```python
from build123d import *

# Parameters (mm, degrees)
SKETCH_1_R          = 4.5
SKETCH_1_R_2        = 1.5
SKETCH_1_W          = 5
SKETCH_1_H          = 9
SKETCH_1_R_3        = 2.5
SKETCH_1_R_4        = 1.1
EXTRUDE_1_DEPTH     = 3
CUT_EXTRUDE_1_DEPTH = 35.179672321


with BuildPart() as part:
    # 草图1 → 凸台-拉伸1 (new body)
    # profile 1 of 12: a face of its own
    with BuildSketch(Plane(origin=(0, 0, 0), x_dir=(1, 0, 0), z_dir=(0, 1, 0))):
        with Locations((-25, 0)):
            Circle(SKETCH_1_R)
        with Locations(Location((-25, 0, 0), (0, 0, 270))):
            Circle(SKETCH_1_R_2, mode=Mode.SUBTRACT)
    # profile 2 of 12: a face of its own
    with BuildSketch(Plane(origin=(0, 0, 0), x_dir=(1, 0, 0), z_dir=(0, 1, 0))):
        with BuildLine():
            Line((-18.5, 4.5), (-25, 4.5))
            ThreePointArc((-25, 4.5), (-21.818019485, 3.181980515), (-20.5, 0))
            ThreePointArc((-20.5, 0), (-21.818019485, -3.181980515), (-25, -4.5))
            Line((-25, -4.5), (-18.5, -4.5))
            Line((-18.5, -4.5), (-18.5, 4.5))
        make_face()
    # profile 3 of 12: a face of its own
    with BuildSketch(Plane(origin=(0, 0, 0), x_dir=(1, 0, 0), z_dir=(0, 1, 0))):
        with Locations((-16, 0)):
            Rectangle(SKETCH_1_W, SKETCH_1_H)
    # profile 4 of 12: a face of its own
    with BuildSketch(Plane(origin=(0, 0, 0), x_dir=(1, 0, 0), z_dir=(0, 1, 0))):
        with BuildLine():
            Line((-13.5, -4.5), (-18.5, -4.5))
            Line((-18.5, -4.5), (-18.5, -15.7))
            Line((-18.5, -15.7), (-7.000000018, -15.7))
            ThreePointArc((-7.000000018, -15.7), (-9.5, -13.199999991), (-7, -10.7))
            Line((-7, -10.7), (-13.5, -10.7))
            Line((-13.5, -10.7), (-13.5, -4.5))
        make_face()
    # profile 5 of 12: a face of its own
    with BuildSketch(Plane(origin=(0, 0, 0), x_dir=(1, 0, 0), z_dir=(0, 1, 0))):
        with BuildLine():
            Line((4.5, -4.5), (-0.5, -4.5))
            Line((-0.5, -4.5), (-0.5, -10.7))
            Line((-0.5, -10.7), (-7, -10.7))
            ThreePointArc((-7, -10.7), (-5.232233047, -11.432233047), (-4.5, -13.2))
            ThreePointArc((-4.5, -13.2), (-5.232233054, -14.967766959), (-7.000000018, -15.7))
            Line((-7.000000018, -15.7), (4.5, -15.7))
            Line((4.5, -15.7), (4.5, -4.5))
        make_face()
    # profile 6 of 12: a face of its own
    with BuildSketch(Plane(origin=(0, 0, 0), x_dir=(1, 0, 0), z_dir=(0, 1, 0))):
        Polygon((4.5, 4.5), (-0.5, 4.5), (-0.5, -4.5), (4.5, -4.5), (4.5, 0), align=None)
    # profile 7 of 12: a face of its own
    with BuildSketch(Plane(origin=(0, 0, 0), x_dir=(1, 0, 0), z_dir=(0, 1, 0))):
        with BuildLine():
            Line((-0.5, 12), (-0.5, 4.5))
            Line((-0.5, 4.5), (4.5, 4.5))
            Line((4.5, 4.5), (4.5, 17))
            Line((4.5, 17), (-7.000000057, 17))
            ThreePointArc((-7.000000057, 17), (-5.232233067, 16.267766973), (-4.5, 14.5))
            ThreePointArc((-4.5, 14.5), (-5.232233047, 12.732233047), (-7, 12))
            Line((-7, 12), (-0.5, 12))
        make_face()
    # profile 8 of 12: a face of its own
    with BuildSketch(Plane(origin=(0, 0, 0), x_dir=(1, 0, 0), z_dir=(0, 1, 0))):
        with BuildLine():
            Line((-18.5, 17), (-18.5, 4.5))
            Line((-18.5, 4.5), (-13.5, 4.5))
            Line((-13.5, 4.5), (-13.5, 12))
            Line((-13.5, 12), (-7, 12))
            ThreePointArc((-7, 12), (-9.5, 14.499999972), (-7.000000057, 17))
            Line((-7.000000057, 17), (-18.5, 17))
        make_face()
    # profile 9 of 12: a face of its own
    with BuildSketch(Plane(origin=(0, 0, 0), x_dir=(1, 0, 0), z_dir=(0, 1, 0))):
        with BuildLine():
            Line((25, 4.5), (4.5, 4.5))
            Line((4.5, 4.5), (4.5, 0))
            Line((4.5, 0), (4.5, -4.5))
            Line((4.5, -4.5), (25, -4.5))
            ThreePointArc((25, -4.5), (20.5, 0), (25, 4.5))
        make_face()
    # profile 10 of 12: a face of its own
    with BuildSketch(Plane(origin=(0, 0, 0), x_dir=(1, 0, 0), z_dir=(0, 1, 0))):
        with Locations((25, 0)):
            Circle(SKETCH_1_R)
        with Locations(Location((25, 0, 0), (0, 0, 270))):
            Circle(SKETCH_1_R_2, mode=Mode.SUBTRACT)
    # profile 11 of 12: a face of its own
    with BuildSketch(Plane(origin=(0, 0, 0), x_dir=(1, 0, 0), z_dir=(0, 1, 0))):
        with Locations((-7, 14.5)):
            Circle(SKETCH_1_R_3)
        with Locations(Location((-7, 14.5, 0), (0, 0, 270))):
            Circle(SKETCH_1_R_4, mode=Mode.SUBTRACT)
    # profile 12 of 12: a face of its own
    with BuildSketch(Plane(origin=(0, 0, 0), x_dir=(1, 0, 0), z_dir=(0, 1, 0))):
        with Locations((-7, -13.2)):
            Circle(SKETCH_1_R_3)
        with Locations(Location((-7, -13.2, 0), (0, 0, 270))):
            Circle(SKETCH_1_R_4, mode=Mode.SUBTRACT)
    extrude(amount=EXTRUDE_1_DEPTH)

    # 草图2 → 切除-拉伸1 (cut, through all)
    with BuildSketch(Plane(origin=(0, 3, 0), x_dir=(1, 0, 0), z_dir=(0, 1, 0))):
        Polygon((4.5, -15.7), (4.5, -11.296015474), (-4.064964363, -15.7), align=None)
    extrude(amount=-CUT_EXTRUDE_1_DEPTH, mode=Mode.SUBTRACT)


solid = part.part
```
Check sheet for the modelled part. Datum: model origin and axes. Units: mm. A direction names the side the tool comes from. Coordinates: 2 decimals unless noted, no trailing zeros. Write each loop counter-clockwise with the first axis right and the second up, starting at its lowest first coordinate (ties: lowest second). Pieces come first, ordered by that corner, then holes. Notation, with made-up numbers: (44, -16.75) -> (56, -16.75) arc R24 ccw to (56, 4.25) -> close; hole circle Ø5 at (37.5, 55.25). An arc over 180 degrees is marked (long way). Use a Markdown table: item, result.
1. Sectioned sample at C-C (x = -7). Enter the section's corners in (y, z), plus the area to 3 significant figures.
Reported:
| item | result |
|---|---|
| outline | (0, -17) -> (3, -17) -> (3, -15.6) -> (0, -15.6) -> close; (0, -13.4) -> (3, -13.4) -> (3, -12) -> (0, -12) -> close; (0, 10.7) -> (3, 10.7) -> (3, 12.1) -> (0, 12.1) -> close; (0, 14.3) -> (3, 14.3) -> (3, 15.7) -> (0, 15.7) -> close |
| area | 16.8 mm2 |
2. Scan lines: line 1 along X through (y, z) = (0.5, 8); line 2 along X through (y, z) = (1.6, 0); line 3 along Z through (x, y) = (-12.5, 2.3). Record each from-to range of solid material in increasing order.
Reported:
| item | result |
|---|---|
| line 1 | x = -18.5 to -13.5, -0.5 to 4.5 |
| line 2 | x = -29.5 to -26.5, -23.5 to -13.5, -0.5 to 23.5, 26.5 to 29.5 |
| line 3 | z = -17 to -12, 10.7 to 15.7 |
3. Tool access check on faces 5 (the flat face through (4.5, 1, -11)), 6 (the flat face through (-7, 1, 10.7)), 7 (the flat face through (-22, 1, 4.5)), 8 (the flat face through (-22, 1, -4.5)). Record the directions out of +Z, -Z, +X, -X, +Y, -Y that give a thin tool (end or side, any length) a straight path to the whole face; none if there is none.
Reported:
| item | result |
|---|---|
| face 5 | -Z, +X, +Y, -Y |
| face 6 | +Y, -Y |
| face 7 | +Z, -X, +Y, -Y |
| face 8 | -Z, -X, +Y, -Y |
4. Sectioned sample at D-D (z = 0). Enter the section's corners in (x, y).
Reported:
| item | result |
|---|---|
| outline | (-29.5, 0) -> (-26.5, 0) -> (-26.5, 3) -> (-29.5, 3) -> close; (-23.5, 0) -> (-13.5, 0) -> (-13.5, 3) -> (-23.5, 3) -> close; (-0.5, 0) -> (23.5, 0) -> (23.5, 3) -> (-0.5, 3) -> close; (26.5, 0) -> (29.5, 0) -> (29.5, 3) -> (26.5, 3) -> close |
5. Release check for a two-part mould opening along Z. For faces 1 (the flat face through (-18.5, 1, 10)), 2 (the flat face through (-0.5, 1, -1)), 3 (the cylindrical face through (-23.513, 1.479, -0.195)), 4 (the cylindrical face through (29.5, 1.5, 0.1)) record: pulls with the +Z half, pulls with the -Z half, needs draft (parallel to the pull), parting line crosses it, or undercut.
Reported:
| item | result |
|---|---|
| face 1 | needs draft |
| face 2 | undercut |
| face 3 | undercut |
| face 4 | parting line crosses it |
6. Sectioned sample at B-B (y = 1.45). Enter the section's corners in (x, z), plus the area to 3 significant figures.
Reported:
| item | result |
|---|---|
| outline | (-25, -4.5) -> (-18.5, -4.5) -> (-18.5, -17) -> (4.5, -17) -> (4.5, -4.5) -> (25, -4.5) arc R4.5 ccw to (25, 4.5) -> (4.5, 4.5) -> (4.5, 11.3) -> (-4.06, 15.7) -> (-18.5, 15.7) -> (-18.5, 4.5) -> (-25, 4.5) arc R4.5 ccw to start; hole circle Ø3 at (-25, 0); hole (-13.5, -12) -> (-0.5, -12) -> (-0.5, 10.7) -> (-13.5, 10.7) -> close; hole circle Ø2.2 at (-7, -14.5); hole circle Ø2.2 at (-7, 13.2); hole circle Ø3 at (25, 0) |
| area | 723 mm2 |
7. Go/stop test with flat-tipped pins: pin 1 Ø1.5 at (y, z) = (1.5, -4) entering from -X; pin 2 Ø1.5 at (x, y) = (17, 2) entering from -Z; pin 3 Ø1.5 at (y, z) = (1.5, -12) entering from +X; pin 4 Ø2.5 at (x, z) = (-25, 0) entering from +Y. Record where each tip stops, or that it passes through.
Reported:
| item | result |
|---|---|
| pin 1 | stops at x = -28.11 |
| pin 2 | stops at z = -4.5 |
| pin 3 | stops at x = 4.5 |
| pin 4 | passes through |
8. Sectioned sample at A-A (z = -10). Enter the section's corners in (x, y).
Reported:
| item | result |
|---|---|
| outline | (-18.5, 0) -> (-13.5, 0) -> (-13.5, 3) -> (-18.5, 3) -> close; (-0.5, 0) -> (4.5, 0) -> (4.5, 3) -> (-0.5, 3) -> close |
